Build history of the part. All positions in model axes, mm. A direction names the side the tool comes from. Give positions to 0.01 mm unless a question says otherwise; leave off trailing zeros. Write each loop counter-clockwise with the first axis right and the second up, starting at its lowest first coordinate (ties: lowest second). Pieces come first, ordered by that corner, then holes. Notation, with made-up numbers: (0, 10) -> (54, 10) arc R13 ccw to (54, 26) -> close; hole circle Ø7 at (71, -31). An arc over 180 degrees is marked (long way). Write item = value, one per line. Start each with the question number.
Q1. Wall check: line 1 (X direction, y = 3.5, z = 7); line 2 (X direction, y = -15, z = -4); line 3 (Y direction, x = 3, z = 4). Give the ranges that are in metal, low to high.
Q2. Saw through at C-C, the plane z = -34.5. List the corners of the cut face in (x, y), then the cut area to 3 significant figures.
Q3. Drop flat-ended pins along their axis: P1, Ø8, axis at y = -9, z = 9, coming from the -X side; P2, Ø2, axis at x = 56, y = -9.5, coming from the +Z side; P3, Ø4, axis at y = 7.5, z = 0.5, coming from the +X side; P4, Ø6, axis at x = 37, z = -2, coming from the -Y side. Give the stop position or say it passes through.
Q4. Mould opens along Y. For faces 5 (the face through (-95.1, -18, -34)), 6 (the face through (0, 23, 2)), 7 (the face through (42, 21.2, 7)) say: pulls with the +Y half, pulls with the -Y half, needs draft (parallel to the pull), parting line crosses it, or undercut.
Q5. Tool access for faces 1 (the face through (-21.2, 0, 7)), 2 (the face through (-19, 0, 0)), 3 (the face through (-42, 17.2, 1)), 4 (the face through (-53.5, 0, -34)): list every direction of +Z, -Z, +X, -X, +Y, -Y with a clear straight run to the whole face (end or side of a thin tool).
Q6. Saw through at B-B, the plane y = -19. Give the number of separate pieces and of enclosed holes in the cut face, then the cut area to 3 significant figures.
Q7. Saw through at A-A, the plane x = -15. List the corners of the cut face in (y, z), then the cut area to 3 significant figures.
from build123d import *

# Parameters (mm, degrees)
SKETCH_W      = 127
SKETCH_H      = 46
PAD_DEPTH     = 2
SKETCH001_W   = 127
SKETCH001_H   = 46
SKETCH001_W_2 = 42.4
SKETCH001_H_2 = 42.4
SKETCH001_W_3 = 38.7
PAD001_DEPTH  = 10
SKETCH002_W   = 24.5
SKETCH002_H   = 34.4
SKETCH002_W_2 = 34.4
POCKET_DEPTH  = 2.001
SKETCH004_W   = 12
SKETCH004_H   = 46
PAD002_DEPTH  = 30.5
PAD003_DEPTH  = 8
FILLET_R      = 10


with BuildPart() as part:
    # Sketch → Pad (new body)
    with BuildSketch(Plane.XY):
        Rectangle(SKETCH_W, SKETCH_H)
    extrude(amount=PAD_DEPTH)

    # Sketch001 → Pad001 (new body)
    with BuildSketch(Plane.XY.offset(2)):
        Rectangle(SKETCH001_W, SKETCH001_H)
        Rectangle(SKETCH001_W_2, SKETCH001_H_2, mode=Mode.SUBTRACT)
        with Locations((-42.35, 0)):
            Rectangle(SKETCH001_W_3, SKETCH001_H_2, mode=Mode.SUBTRACT)
        with Locations((42.35, 0)):
            Rectangle(SKETCH001_W_3, SKETCH001_H_2, mode=Mode.SUBTRACT)
    extrude(amount=PAD001_DEPTH)

    # Sketch002 → Pocket (cut, through all)
    with BuildSketch(Plane.XY.offset(2)):
        with Locations((-39.25, 0)):
            Rectangle(SKETCH002_W, SKETCH002_H)
        Rectangle(SKETCH002_W_2, SKETCH002_H)
        with Locations((39.25, 0)):
            Rectangle(SKETCH002_W, SKETCH002_H)
    extrude(amount=-POCKET_DEPTH, mode=Mode.SUBTRACT)

    # Sketch004 → Pad002 (new body)
    with BuildSketch(Plane(origin=(0, 0, 0), x_dir=(1, 0, 0), z_dir=(0, 0, -1))):
        with Locations((-57.5, 0)):
            Rectangle(SKETCH004_W, SKETCH004_H)
        with Locations((57.5, 0)):
            Rectangle(SKETCH004_W, SKETCH004_H)
    extrude(amount=PAD002_DEPTH)

    # Sketch005 → Pad003 (new body)
    with BuildSketch(Plane(origin=(0, 0, -30.5), x_dir=(1, 0, 0), z_dir=(0, 0, -1))):
        Polygon((-51.5, 23), (-95.1, 23), (-95.1, 13), (-93.1, 13), (-93.1, 21), (-53.5, 21), (-53.5, -21), (-93.1, -21), (-93.1, -13), (-95.1, -13), (-95.1, -23), (-51.5, -23), align=None)
        Polygon((51.5, 23), (95.1, 23), (95.1, 13), (93.1, 13), (93.1, 21), (53.5, 21), (53.5, -21), (93.1, -21), (93.1, -13), (95.1, -13), (95.1, -23), (51.5, -23), align=None)
    extrude(amount=PAD003_DEPTH)

    # Fillet
    fillet_edges = [part.edges().sort_by_distance(p)[0] for p in [
        (-63.5, -22, -30.5),
        (-63.5, 22, -30.5),
        (63.5, -22, -30.5),
        (63.5, 22, -30.5),
        (-51.5, -20.1, 0),
        (-51.5, 20.1, 0),
        (51.5, -20.1, 0),
        (51.5, 20.1, 0),
    ]]
    fillet(fillet_edges, radius=FILLET_R)


solid = part.part
Report:
q1.line_1 = -63.5 to -61.7, -23 to -21.2, 21.2 to 23, 61.7 to 63.5
q1.line_2 = -63.5 to -51.5, 51.5 to 63.5
q1.line_3 = -23 to -21.2, 21.2 to 23
q2.outline = (-95.1, -23) -> (-51.5, -23) -> (-51.5, 23) -> (-95.1, 23) -> (-95.1, 13) -> (-93.1, 13) -> (-93.1, 21) -> (-53.5, 21) -> (-53.5, -21) -> (-93.1, -21) -> (-93.1, -13) -> (-95.1, -13) -> close; (51.5, -23) -> (95.1, -23) -> (95.1, -13) -> (93.1, -13) -> (93.1, -21) -> (53.5, -21) -> (53.5, 21) -> (93.1, 21) -> (93.1, 13) -> (95.1, 13) -> (95.1, 23) -> (51.5, 23) -> close
q2.area = 581 mm2
q3.P1 = -63.5
q3.P2 = 2
q3.P3 = 63.5
q3.P4 = -23
q4.face_5 = needs draft
q4.face_6 = pulls with the +Y half
q4.face_7 = undercut
q5.face_1 = +Z
q5.face_2 = -Z, +Y, -Y
q5.face_3 = +Z, -Z
q5.face_4 = -Z
q6.separate_pieces = 3
q6.enclosed_holes = 0
q6.area = 1,160 mm2
q7.outline = (-23, 0) -> (-17.2, 0) -> (-17.2, 2) -> (-21.2, 2) -> (-21.2, 12) -> (-23, 12) -> close; (17.2, 0) -> (23, 0) -> (23, 12) -> (21.2, 12) -> (21.2, 2) -> (17.2, 2) -> close
q7.area = 59.2 mm2
